from build123d import *

# Parameters (mm, degrees)
SKETCH1_W                        = 609.6
SKETCH1_H                        = 609.6
BOSS_EXTRUDE1_DEPTH              = 2.65684
CUT_EXTRUDE1_DEPTH               = 3.65684
SKETCH3_R                        = 2.3876
CUT_EXTRUDE2_DEPTH               = 3.65684
LPATTERN1_COUNT                  = 2
LPATTERN1_PITCH                  = 203.2
CUT_EXTRUDE3_DEPTH               = 3.65684
FILLET1_R                        = 12.7
SKETCH5_R                        = 2.3876
CUT_EXTRUDE4_DEPTH               = 3.65684
F_10_0_1935_DIAMETER_HOLE1_D     = 4.9149
F_10_0_1935_DIAMETER_HOLE1_DEPTH = 2.65684


with BuildPart() as part:
    # Sketch1 → Boss-Extrude1 (new body)
    with BuildSketch(Plane(origin=(0, 0, 0), x_dir=(1, 0, 0), z_dir=(0, 1, 0))):
        Rectangle(SKETCH1_W, SKETCH1_H)
    extrude(amount=BOSS_EXTRUDE1_DEPTH)

    # Sketch2 → Cut-Extrude1 (cut, through all)
    with BuildSketch(Plane(origin=(0, 2.65684, 0), x_dir=(1, 0, 0), z_dir=(0, 1, 0))):
        with BuildLine():
            Line((-104.775, 123.825), (-66.675, 123.825))
            ThreePointArc((-66.675, 123.825), (-62.184871939, 121.965128061), (-60.325, 117.475))
            Line((-60.325, 117.475), (-60.325, 53.975))
            ThreePointArc((-60.325, 53.975), (-62.184871939, 49.484871939), (-66.675, 47.625))
            Line((-66.675, 47.625), (-104.775, 47.625))
            ThreePointArc((-104.775, 47.625), (-109.265128061, 49.484871939), (-111.125, 53.975))
            Line((-111.125, 53.975), (-111.125, 117.475))
            ThreePointArc((-111.125, 117.475), (-109.265128061, 121.965128061), (-104.775, 123.825))
        make_face()
        with BuildLine():
            Line((-104.775, -47.625), (-66.675, -47.625))
            ThreePointArc((-66.675, -47.625), (-62.184871939, -49.484871939), (-60.325, -53.975))
            Line((-60.325, -53.975), (-60.325, -117.475))
            ThreePointArc((-60.325, -117.475), (-62.184871939, -121.965128061), (-66.675, -123.825))
            Line((-66.675, -123.825), (-104.775, -123.825))
            ThreePointArc((-104.775, -123.825), (-109.265128061, -121.965128061), (-111.125, -117.475))
            Line((-111.125, -117.475), (-111.125, -53.975))
            ThreePointArc((-111.125, -53.975), (-109.265128061, -49.484871939), (-104.775, -47.625))
        make_face()
        with BuildLine():
            Line((66.675, -47.625), (104.775, -47.625))
            ThreePointArc((104.775, -47.625), (109.265128061, -49.484871939), (111.125, -53.975))
            Line((111.125, -53.975), (111.125, -117.475))
            ThreePointArc((111.125, -117.475), (109.265128061, -121.965128061), (104.775, -123.825))
            Line((104.775, -123.825), (66.675, -123.825))
            ThreePointArc((66.675, -123.825), (62.184871939, -121.965128061), (60.325, -117.475))
            Line((60.325, -117.475), (60.325, -53.975))
            ThreePointArc((60.325, -53.975), (62.184871939, -49.484871939), (66.675, -47.625))
        make_face()
        with BuildLine():
            Line((104.775, 123.825), (66.675, 123.825))
            ThreePointArc((66.675, 123.825), (62.184871939, 121.965128061), (60.325, 117.475))
            Line((60.325, 117.475), (60.325, 53.975))
            ThreePointArc((60.325, 53.975), (62.184871939, 49.484871939), (66.675, 47.625))
            Line((66.675, 47.625), (104.775, 47.625))
            ThreePointArc((104.775, 47.625), (109.265128061, 49.484871939), (111.125, 53.975))
            Line((111.125, 53.975), (111.125, 117.475))
            ThreePointArc((111.125, 117.475), (109.265128061, 121.965128061), (104.775, 123.825))
        make_face()
    extrude(amount=-CUT_EXTRUDE1_DEPTH, mode=Mode.SUBTRACT)

    # Sketch3 → Cut-Extrude2 (cut, through all)
    with BuildSketch(Plane(origin=(0, 2.65684, 0), x_dir=(1, 0, 0), z_dir=(0, 1, 0))):
        with Locations((-165.1, 127)):
            Circle(SKETCH3_R)
        with Locations((-165.1, 0)):
            Circle(SKETCH3_R)
        with Locations((-165.1, -127)):
            Circle(SKETCH3_R)
        with Locations((-38.1, 127)):
            Circle(SKETCH3_R)
        with Locations((-38.1, 0)):
            Circle(SKETCH3_R)
        with Locations((-38.1, -127)):
            Circle(SKETCH3_R)
    cut_extrude2 = extrude(amount=-CUT_EXTRUDE2_DEPTH, mode=Mode.SUBTRACT)

    # LPattern1: Cut-Extrude2 ×2
    with Locations(*[(i * LPATTERN1_PITCH, 0, 0) for i in range(1, LPATTERN1_COUNT)]):
        add(cut_extrude2, mode=Mode.SUBTRACT)

    # Sketch4 → Cut-Extrude3 (cut, through all)
    with BuildSketch(Plane(origin=(0, 2.65684, 0), x_dir=(1, 0, 0), z_dir=(0, 1, 0))):
        with BuildLine():
            Line((-63.5, -238.125), (63.5, -238.125))
            ThreePointArc((63.5, -238.125), (79.375, -254), (63.5, -269.875))
            Line((63.5, -269.875), (-63.5, -269.875))
            ThreePointArc((-63.5, -269.875), (-79.375, -254), (-63.5, -238.125))
        make_face()
    extrude(amount=-CUT_EXTRUDE3_DEPTH, mode=Mode.SUBTRACT)

    # Fillet1
    fillet1_edges = [part.edges().sort_by_distance(p)[0] for p in [
        (304.8, 1.32842, 304.8),
        (-304.8, 1.32842, 304.8),
        (-304.8, 1.32842, -304.8),
        (304.8, 1.32842, -304.8),
    ]]
    fillet(fillet1_edges, radius=FILLET1_R)

    # Sketch5 → Cut-Extrude4 (cut, through all)
    with BuildSketch(Plane(origin=(0, 2.65684, 0), x_dir=(1, 0, 0), z_dir=(0, 1, 0))):
        with Locations((161.925, 292.1)):
            Circle(SKETCH5_R)
        with Locations((66.675, 292.1)):
            Circle(SKETCH5_R)
        with Locations((161.925, 193.675)):
            Circle(SKETCH5_R)
        with Locations((66.675, 193.675)):
            Circle(SKETCH5_R)
        with Locations((193.675, 161.925)):
            Circle(SKETCH5_R)
        with Locations((193.675, 66.675)):
            Circle(SKETCH5_R)
        with Locations((292.1, 66.675)):
            Circle(SKETCH5_R)
        with Locations((292.1, 161.925)):
            Circle(SKETCH5_R)
    extrude(amount=-CUT_EXTRUDE4_DEPTH, mode=Mode.SUBTRACT)

    # #10 (0.1935) Diameter Hole1
    with Locations(Plane(origin=(0, 2.65684, 0), x_dir=(1, 0, 0), z_dir=(0, 1, 0))):
        with Locations((161.925, 292.1), (66.675, 292.1), (292.1, 161.925), (193.675, 161.925), (161.925, 193.675), (66.675, 193.675), (165.1, 127), (38.1, 127), (-38.1, 127), (292.1, 66.675), (193.675, 66.675), (165.1, 0), (165.1, -127), (-38.1, 0), (38.1, 0), (38.1, -127), (-38.1, -127), (-165.1, -127), (-165.1, 0), (-165.1, 127)):
            Hole(F_10_0_1935_DIAMETER_HOLE1_D / 2, depth=F_10_0_1935_DIAMETER_HOLE1_DEPTH)


solid = part.part
Geometry check sheet. Reference: the model listing, model coordinates, mm. A direction names the side the tool comes from. Give positions to 0.01 mm unless a question says otherwise; leave off trailing zeros. Loops run counter-clockwise (first coordinate to the right, second up) from the corner with the lowest first, then second, coordinate; pieces in that order, holes last. Notation, with made-up numbers: M 87.5,37.25 L 98.5,37.25 A20 cw 98.5,66.25 Z; hole C -18.75,52.5 d3. An arc over 180 degrees is marked long. Write each question's results on one line, items separated by ' | '.
1) Thickness scan on line 1 (Z direction, x = 102, y = 0.3) (3 decimals); line 2 (X direction, y = 1.9, z = -127); line 3 (Z direction, x = -165.1, y = 1.75). Record the ranges inside material, lowest first.
Answers follow:
line 1: -304.8 to -123.825, -47.625 to 47.625, 123.825 to 304.8 | line 2: -304.8 to -167.56, -162.64 to -40.56, -35.64 to 35.64, 40.56 to 162.64, 167.56 to 304.8 | line 3: -304.8 to -129.46, -124.54 to -2.46, 2.46 to 124.54, 129.46 to 304.8
2) Section check B-B, the plane z = -106. Record the boundary of the cut face in (x, y) (3 decimals), plus the area to 3 significant figures.
Answers follow:
outline: M -304.8,0 L -111.125,0 L -111.125,2.657 L -304.8,2.657 Z; M -60.325,0 L 60.325,0 L 60.325,2.657 L -60.325,2.657 Z; M 111.125,0 L 304.8,0 L 304.8,2.657 L 111.125,2.657 Z | area: 1,350 mm2
3) Tool access check on faces 1 (the face through (-4, 0, -4)), 2 (the face through (-79.37, 1.35, 254.35)). Record the directions out of +Z, -Z, +X, -X, +Y, -Y that give a thin tool (end or side, any length) a straight path to the whole face; none if there is none.
Answers follow:
face 1: +Z, -Z, +X, -X, -Y | face 2: +Y, -Y
4) Section check A-A, the plane x = 7.5. Record the boundary of the cut face in (y, z) (3 decimals).
Answers follow:
outline: M 0,-304.8 L 2.657,-304.8 L 2.657,238.125 L 0,238.125 Z; M 0,269.875 L 2.657,269.875 L 2.657,304.8 L 0,304.8 Z
5) Section check D-D, the plane y = 2. Count the separate pieces of the cut face and the enclosed holes in it, plus the area to 3 significant figures.
Answers follow:
separate pieces: 1 | enclosed holes: 25 | area: 351,000 mm2
6) Section check C-C, the plane x = 89. Record the boundary of the cut face in (y, z) (3 decimals).
Answers follow:
outline: M 0,-304.8 L 2.657,-304.8 L 2.657,-123.825 L 0,-123.825 Z; M 0,-47.625 L 2.657,-47.625 L 2.657,47.625 L 0,47.625 Z; M 0,123.825 L 2.657,123.825 L 2.657,304.8 L 0,304.8 Z
7) Release check for a two-part mould opening along Z. For faces 3 (the face through (79.37, 1.35, 253.65)), 4 (the face through (-4, 2.657, -4)) record: +Z half, -Z half, draft (parallel to the pull), parting line (faces both ways), or undercut.
Answers follow:
face 3: undercut | face 4: draft
